```python
from build123d import *

# Parameters (mm, degrees)
CYLINDER009_R     = 4
CYLINDER009_DEPTH = 10
CYLINDER008_R     = 4
CYLINDER008_DEPTH = 10
CYLINDER002_R     = 1.5
CYLINDER002_DEPTH = 25
ARRAY002_COUNT    = 4
CYLINDER003_R     = 11
CYLINDER003_DEPTH = 10
CYLINDER005_R     = 11
CYLINDER005_DEPTH = 5
CYLINDER004_R     = 4
CYLINDER004_DEPTH = 30
CYLINDER_R        = 2
CYLINDER_DEPTH    = 25
ARRAY_Y_COUNT     = 2
ARRAY_Y_PITCH     = 50
CYLINDER001_R     = 2
CYLINDER001_DEPTH = 25
ARRAY001_X_COUNT  = 2
ARRAY001_X_PITCH  = 16
BOX_W             = 150
BOX_H             = 70
BOX_DEPTH         = 18
BOX001_W          = 11
BOX001_H          = 6
BOX001_DEPTH      = 25
CYLINDER006_R     = 3
CYLINDER006_DEPTH = 25
CYLINDER007_R     = 3
CYLINDER007_DEPTH = 25


with BuildPart() as cilindro009:
    # Cylinder009 → Cylinder009 (new body)
    with BuildSketch(Plane(origin=(240, 61, 0), x_dir=(1, 0, 0), z_dir=(0, 0, 1))):
        Circle(CYLINDER009_R)
    extrude(amount=CYLINDER009_DEPTH)


with BuildPart() as cilindro008:
    # Cylinder008 → Cylinder008 (new body)
    with BuildSketch(Plane(origin=(60, 61, 0), x_dir=(1, 0, 0), z_dir=(0, 0, 1))):
        Circle(CYLINDER008_R)
    extrude(amount=CYLINDER008_DEPTH)


with BuildPart() as array002:
    # Cylinder002 → Cylinder002 (new body)
    with BuildSketch(Plane(origin=(22, 0, 0), x_dir=(1, 0, 0), z_dir=(0, 0, 1))):
        Circle(CYLINDER002_R)
    extrude(amount=CYLINDER002_DEPTH)

    # Array002: Array002 ×4 about axis
    array002_axis = Axis((0, 0, 0), (0, 0, 1))


with BuildPart() as array002_1:
    add(array002.part)
    for i in range(1, ARRAY002_COUNT):
        add(array002.part.rotate(array002_axis, i * 360 / ARRAY002_COUNT))


with BuildPart() as array002_2:
    # Array002 placement: moved
    add(array002_1.part.moved(Location((150, 60, 0))))


with BuildPart() as cilindro003:
    # Cylinder003 → Cylinder003 (new body)
    with BuildSketch(Plane.XY.offset(15)):
        Circle(CYLINDER003_R)
    extrude(amount=CYLINDER003_DEPTH)


with BuildPart() as fusion:
    # Cylinder005 → Cylinder005 (new body)
    with BuildSketch(Plane.XY):
        Circle(CYLINDER005_R)
    extrude(amount=CYLINDER005_DEPTH)

    # Fusion: union Cilindro003
    add(cilindro003.part)


with BuildPart() as fusion_1:
    # Fusion placement: moved
    add(fusion.part.moved(Location((150, 60, 0))))


with BuildPart() as huecomotor:
    # Cylinder004 → Cylinder004 (new body)
    with BuildSketch(Plane(origin=(150, 60, 0), x_dir=(1, 0, 0), z_dir=(0, 0, 1))):
        Circle(CYLINDER004_R)
    extrude(amount=CYLINDER004_DEPTH)

    # Fusion001: union Fusion
    add(fusion_1.part)


with BuildPart() as array:
    # Cylinder → Cylinder (new body)
    with BuildSketch(Plane.XY):
        Circle(CYLINDER_R)
    extrude(amount=CYLINDER_DEPTH)

    # Array Y: Array ×2


with BuildPart() as array_1:
    add(array.part)
    with Locations(*[(0, i * ARRAY_Y_PITCH, 0) for i in range(1, ARRAY_Y_COUNT)]):
        add(array.part)


with BuildPart() as array_2:
    # Array placement: moved
    add(array_1.part.moved(Location((9, 10, 0))))


with BuildPart() as array001:
    # Cylinder001 → Cylinder001 (new body)
    with BuildSketch(Plane(origin=(28, 0, 0), x_dir=(1, 0, 0), z_dir=(0, 0, 1))):
        Circle(CYLINDER001_R)
    extrude(amount=CYLINDER001_DEPTH)

    # Array001 X: Array001 ×2


with BuildPart() as array001_1:
    add(array001.part)
    with Locations(*[(i * ARRAY001_X_PITCH, 0, 0) for i in range(1, ARRAY001_X_COUNT)]):
        add(array001.part)


with BuildPart() as array001_2:
    # Array001 placement: moved
    add(array001_1.part.moved(Location((0, 35, 0))))


with BuildPart() as base:
    # Box → Box (new body)
    with BuildSketch(Plane.XY):
        with Locations((75, 35)):
            Rectangle(BOX_W, BOX_H)
    extrude(amount=BOX_DEPTH)

    # Cut: cut Array001
    add(array001_2.part, mode=Mode.SUBTRACT)

    # Cut001: cut Array
    add(array_2.part, mode=Mode.SUBTRACT)


with BuildPart() as mirror_of_base:
    # mirror: instance of Base
    add(base.part.mirror(Plane(origin=(150, 0, 0), x_dir=(0, 1, 0), z_dir=(-1, 0, 0))))


with BuildPart() as cubo001:
    # Box001 → Box001 (new body)
    with BuildSketch(Plane(origin=(120, 27, 0), x_dir=(1, 0, 0), z_dir=(0, 0, 1))):
        with Locations((5.5, 3)):
            Rectangle(BOX001_W, BOX001_H)
    extrude(amount=BOX001_DEPTH)


with BuildPart() as cilindro006:
    # Cylinder006 → Cylinder006 (new body)
    with BuildSketch(Plane(origin=(120, 30, 0), x_dir=(1, 0, 0), z_dir=(0, 0, 1))):
        Circle(CYLINDER006_R)
    extrude(amount=CYLINDER006_DEPTH)


with BuildPart() as fusion002:
    # Cylinder007 → Cylinder007 (new body)
    with BuildSketch(Plane(origin=(131, 30, 0), x_dir=(1, 0, 0), z_dir=(0, 0, 1))):
        Circle(CYLINDER007_R)
    extrude(amount=CYLINDER007_DEPTH)

    # Fusion002: union Cubo001, Cilindro006
    add(cubo001.part)
    add(cilindro006.part)


with BuildPart() as cut006:
    # Cut002 base: copy of Base
    add(base.part)

    # Cut002: cut Fusion002
    add(fusion002.part, mode=Mode.SUBTRACT)

    # Fusion003: union Mirror of Base
    add(mirror_of_base.part)

    # Cut003: cut HuecoMotor
    add(huecomotor.part, mode=Mode.SUBTRACT)

    # Cut004: cut Array002
    add(array002_2.part, mode=Mode.SUBTRACT)

    # Cut005: cut Cilindro008
    add(cilindro008.part, mode=Mode.SUBTRACT)

    # Cut006: cut Cilindro009
    add(cilindro009.part, mode=Mode.SUBTRACT)


solid = cut006.part
```
Can you work these out from the model? Positions are in its coordinate system, mm. A direction names the side the tool comes from. Round coordinates to 2 decimals unless told otherwise and drop trailing zeros. Loops run counter-clockwise (first coordinate to the right, second up) from the corner with the lowest first, then second, coordinate; pieces in that order, holes last. Notation, with made-up numbers: M -22.5,58.5 L -17.5,58.5 A28 cw -17.5,84.5 Z; hole C -1.5,-21 d3. An arc over 180 degrees is marked long. Answer in a Markdown table with one row per item.
1. On a 3-axis mill with a long thin cutter (end or side, diameter ignored), from which of +Z, -Z, +X, -X, +Y, -Y can I reach the whole of each face in a straight line? I mean faces 4 (the face through (0, 35, 9)), 5 (the face through (117, 30, 9)), 6 (the face through (150, 49, 16)), 7 (the face through (149.8, 64.3, 5)), 8 (the face through (300, 35, 9)). Say none if no direction works.
Established:
| item | result |
|---|---|
| face 4 | +Z, -Z, -X, +Y, -Y |
| face 5 | +Z, -Z |
| face 6 | +Z |
| face 7 | -Z |
| face 8 | +Z, -Z, +X, +Y, -Y |
2. I'm going to push flat-ended pins straight in: pin 1 Ø5 at (x, y) = (150, 60) entering from +Z; pin 2 Ø6.5 at (x, y) = (240, 61) entering from -Z; pin 3 Ø17 at (x, y) = (152, 60.5) entering from +Z. Where does each tip first touch, or does it pass through?
Established:
| item | result |
|---|---|
| pin 1 | through |
| pin 2 | z = 10 |
| pin 3 | z = 15 |
3. Thinking about a two-plate mould opening in Y: for faces 1 (the face through (152, 35, 18)), 2 (the face through (125, 33, 9)), 3 (the face through (152, 0, 9)), which applies, pulls with the +Y half, pulls with the -Y half, needs draft (parallel to the pull), parting line crosses it, or undercut?
Established:
| item | result |
|---|---|
| face 1 | needs draft |
| face 2 | undercut |
| face 3 | pulls with the -Y half |
4. If we section it at B-B, the plane x = 60: Please give me the cut outline in (y, z).
Established:
| item | result |
|---|---|
| outline | M 0,0 L 57,0 L 57,10 L 65,10 L 65,0 L 70,0 L 70,18 L 0,18 Z |
5. Please list where these lines run through material, in increasing order: line 1 (Y direction, x = 150, z = 9); line 2 (X direction, y = 10, z = 4.75); line 3 (Y direction, x = 9, z = 10.5). Write a range as from..to.
Established:
| item | result |
|---|---|
| line 1 | 0..36.5, 39.5..56, 64..70 |
| line 2 | 0..7, 11..289, 293..300 |
| line 3 | 0..8, 12..58, 62..70 |
6. If we section it at C-C, the plane z = 2.5: Give the number of separate pieces and of enclosed holes in the cut face, plus the area to 3 significant figures.
Established:
| item | result |
|---|---|
| separate pieces | 1 |
| enclosed holes | 14 |
| area | 20,300 mm² |
7. If we section it at A-A, the plane y = 30: Please give me the cut outline in (x, z).
Established:
| item | result |
|---|---|
| outline | M 0,0 L 117,0 L 117,18 L 0,18 Z; M 134,0 L 300,0 L 300,18 L 134,18 Z |
